Part model, mm, in its own coordinate system. A direction names the side the tool comes from. Give positions to 0.01 mm unless a question says otherwise; leave off trailing zeros. Order: outer loops, then holes, each group sorted by start corner. A loop starts at its lowest first (then second) coordinate and runs counter-clockwise, first axis right, second up. Notation, with made-up numbers: (53, 47.25) - (90, 47.25) arc R3 ccw to (90, 52.25) - close; hole circle Ø5 at (32.25, 18.25). An arc over 180 degrees is marked (long way). One line per item, written item: value.
```python
from build123d import *
from OCP.BRepFilletAPI import BRepFilletAPI_MakeChamfer

# Parameters (mm, degrees)
FILLET1_R           = 0.2
CUT_EXTRUDE1_START  = -0.1
SKETCH2_R           = 6.5
SKETCH2_R_2         = 4.6
CUT_EXTRUDE1_DEPTH  = 0.1
SKETCH3_W           = 2
SKETCH3_H           = 0.3
SKETCH3_W_2         = 0.3
SKETCH3_H_2         = 2
EXTRUDE_THIN1_DEPTH = 7.6
CHAMFER1_SIZE       = 0.4
CHAMFER1_SIZE2      = 0.692820323


with BuildPart() as part:
    # Sketch1 → Revolve1 (revolve)
    with BuildSketch(Plane(origin=(0, 0, 0), x_dir=(0, 0, -1), z_dir=(1, 0, 0))):
        Polygon((0, 3.4), (-4.6, 3.4), (-4.6, 1.5), (-7, 1.5), (-9, 0.5), (-9, 0), (-8, 0), (-8, -18.6), (-5, -18.6), (-5, -26.4), (0, -26.4), align=None)
    revolve(axis=Axis((0, 14.375, 0), (0, -1, 0)))

    # Fillet1
    fillet1_edges = [part.edges().sort_by_distance(p)[0] for p in [
        (0, 3.4, -4.6),
    ]]
    fillet(fillet1_edges, radius=FILLET1_R)

    # Sketch2 → Cut-Extrude1 (cut)
    with BuildSketch(Plane(origin=(0, 1.5, 0), x_dir=(1, 0, 0), z_dir=(0, 1, 0)).offset(CUT_EXTRUDE1_START)):
        with Locations(Location((0, 0, 0), (0, 0, 270))):
            Circle(SKETCH2_R)
        with Locations(Location((0, 0, 0), (0, 0, 270))):
            Circle(SKETCH2_R_2, mode=Mode.SUBTRACT)
    extrude(amount=CUT_EXTRUDE1_DEPTH, mode=Mode.SUBTRACT)

    # Sketch3 → Extrude-Thin1 (add)
    with BuildSketch(Plane.XZ.offset(26.4)):
        with Locations((0, 4)):
            Rectangle(SKETCH3_W, SKETCH3_H)
        with Locations((0, -4)):
            Rectangle(SKETCH3_W, SKETCH3_H)
        with Locations((-4, 0)):
            Rectangle(SKETCH3_W_2, SKETCH3_H_2)
        with Locations((4, 1)):
            Rectangle(SKETCH3_W_2, SKETCH3_H_2)
    extrude(amount=EXTRUDE_THIN1_DEPTH)

    # Chamfer1: one chamfer whose edges measure the first distance from different faces: ONE call of the kernel's chamfer builder (chamfer() names one face for all edges)
    chamfer1_edges_1 = [part.edges().sort_by_distance(p)[0] for p in [
        (1, -34, 4),
        (-1, -34, 4),
    ]]
    chamfer1_side_1 = [part.faces().sort_by_distance(p)[0] for p in [
        (0, -34, 4),
    ]]
    chamfer1_edges_2 = [part.edges().sort_by_distance(p)[0] for p in [
        (1, -34, -4),
        (-1, -34, -4),
    ]]
    chamfer1_side_2 = [part.faces().sort_by_distance(p)[0] for p in [
        (0, -34, -4),
    ]]
    chamfer1_edges_3 = [part.edges().sort_by_distance(p)[0] for p in [
        (-4, -34, -1),
        (-4, -34, 1),
    ]]
    chamfer1_side_3 = [part.faces().sort_by_distance(p)[0] for p in [
        (-4, -34, 0),
    ]]
    chamfer1_edges_4 = [part.edges().sort_by_distance(p)[0] for p in [
        (4, -34, 2),
        (4, -34, 0),
    ]]
    chamfer1_side_4 = [part.faces().sort_by_distance(p)[0] for p in [
        (4, -34, 1),
    ]]
    chamfer1 = BRepFilletAPI_MakeChamfer(part.part.solid().wrapped)
    for e in chamfer1_edges_1:
        chamfer1.Add(CHAMFER1_SIZE, CHAMFER1_SIZE2, e.wrapped, chamfer1_side_1[0].wrapped)  # the first distance lies on this face
    for e in chamfer1_edges_2:
        chamfer1.Add(CHAMFER1_SIZE, CHAMFER1_SIZE2, e.wrapped, chamfer1_side_2[0].wrapped)  # the first distance lies on this face
    for e in chamfer1_edges_3:
        chamfer1.Add(CHAMFER1_SIZE, CHAMFER1_SIZE2, e.wrapped, chamfer1_side_3[0].wrapped)  # the first distance lies on this face
    for e in chamfer1_edges_4:
        chamfer1.Add(CHAMFER1_SIZE, CHAMFER1_SIZE2, e.wrapped, chamfer1_side_4[0].wrapped)  # the first distance lies on this face
    add(Compound.cast(chamfer1.Shape()), mode=Mode.REPLACE)


solid = part.part
```
1) Drop flat-ended pins along their axis: P1, Ø1.6, axis at y = -29.5, z = -0.5, coming from the -X side; P2, Ø1.5, axis at x = 0.5, z = -1, coming from the -Y side; P3, Ø6, axis at y = -14.5, z = -5, coming from the -X side. Give the stop position or say it passes through.
Answer:
P1: stops at x = -4.15
P2: stops at y = -26.4
P3: stops at x = -7.75
2) Wall check: line 1 along X through (y, z) = (1.45, 0); line 2 along Y through (x, z) = (0.25, 6); line 3 along X through (y, z) = (1.55, 0). Give the ranges that are in metal, low to high. Write a range as [from, to].
Answer:
line 1: x = [-7.1, -6.5], [-4.6, 4.6], [6.5, 7.1]
line 2: y = [-18.6, 1.4]
line 3: x = [-4.6, 4.6]
3) Two-plate mould, pull along Z, no slides. Class faces 1 (the face through (-8.923, 0.246, -1.172)), 2 (the face through (0, -30, -3.85)), 3 (the face through (5.2, -18.6, -0.1)): pulls with the +Z half, pulls with the -Z half, needs draft (parallel to the pull), parting line crosses it, or undercut.
Answer:
face 1: parting line crosses it
face 2: undercut
face 3: needs draft
4) Slice it at B-B on y = -22.5. Write the cut outline in (x, z).
Answer:
outline: circle Ø10 at (0, 0)
5) Slice it at C-C on y = -16. Write the cut outline in (x, z), then the cut area to 3 significant figures.
Answer:
outline: circle Ø16 at (0, 0)
area: 201 mm2
6) Which spindle directions (+Z, -Z, +X, -X, +Y, -Y) get a long thin tool onto all of the face, cutting with end or side? Do faces 4 (the face through (-4, 1.4, 3)), 5 (the face through (-4.15, -30, 0)), 6 (the face through (0, -30, -4.15)). Say none if no direction does.
Answer:
face 4: +Y
face 5: +Z, -Z, -X, -Y
face 6: -Z, +X, -X, -Y
